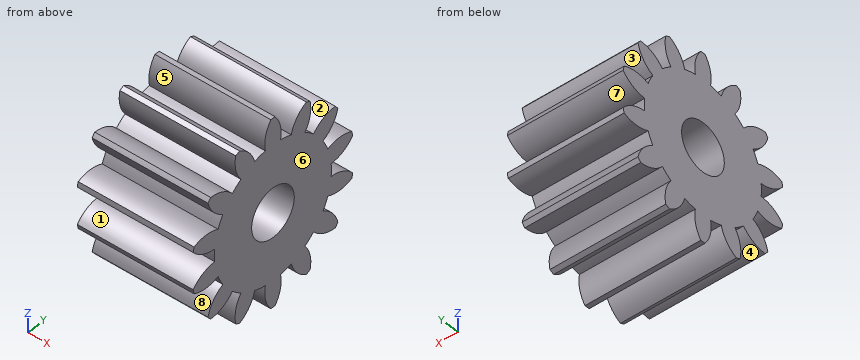
```python
from build123d import *

# Parameters (mm, degrees)
SPUR_START             = 15.199213342
SPUR_GEAR_AM_OUTLINE_R = 2.5
SPUR_GEAR_AM_DEPTH     = 5
SKETCH9_R              = 2.5
SKETCH9_R_2            = 1.05
BOSS_EXTRUDE1_DEPTH    = 5


# Read off the part's stored shape, not the designer's step: spur gear_am
with BuildPart() as part:
    # spur gear_am outline → spur gear_am (new body)
    with BuildSketch(Plane.YZ.offset(SPUR_START)):
        with BuildLine():
            ThreePointArc((2.747947228, -4.643773619), (2.654088149, -4.687486435), (2.561391914, -4.733613923))
            ThreePointArc((2.561391914, -4.733613923), (2.561783739, -5.337982285), (2.816889806, -5.88587111))
            ThreePointArc((2.816889806, -5.88587111), (2.597713415, -6.044378226), (2.394409068, -6.222788256))
            ThreePointArc((2.394409068, -6.222788256), (1.9170234, -5.852161498), (1.327895004, -5.717294884))
            ThreePointArc((1.327895004, -5.717294884), (1.262297175, -5.797402699), (1.198794721, -5.879181519))
            ThreePointArc((1.198794721, -5.879181519), (1.461373347, -6.423528591), (1.928936024, -6.806472991))
            ThreePointArc((1.928936024, -6.806472991), (1.800238579, -7.04438004), (1.694476903, -7.293332374))
            ThreePointArc((1.694476903, -7.293332374), (1.103558354, -7.166539081), (0.514255579, -7.300641692))
            ThreePointArc((0.514255579, -7.300641692), (0.489911456, -7.401278171), (0.468180222, -7.502511024))
            ThreePointArc((0.468180222, -7.502511024), (0.940938733, -7.879022193), (1.528351497, -8.021175333))
            ThreePointArc((1.528351497, -8.021175333), (1.515623105, -8.291361907), (1.528351497, -8.56154848))
            ThreePointArc((1.528351497, -8.56154848), (0.940938733, -8.70370162), (0.468180222, -9.080212789))
            ThreePointArc((0.468180222, -9.080212789), (0.489911456, -9.181445642), (0.514255579, -9.28208212))
            ThreePointArc((0.514255579, -9.28208212), (1.103558354, -9.416184732), (1.694476903, -9.289391439))
            ThreePointArc((1.694476903, -9.289391439), (1.800238579, -9.538343772), (1.928936024, -9.776250821))
            ThreePointArc((1.928936024, -9.776250821), (1.461373347, -10.159195221), (1.198794721, -10.703542294))
            ThreePointArc((1.198794721, -10.703542294), (1.262297175, -10.785321114), (1.327895004, -10.865428928))
            ThreePointArc((1.327895004, -10.865428928), (1.9170234, -10.730562315), (2.394409068, -10.359935556))
            ThreePointArc((2.394409068, -10.359935556), (2.597713414, -10.538345587), (2.816889806, -10.696852703))
            ThreePointArc((2.816889806, -10.696852703), (2.561783739, -11.244741528), (2.561391914, -11.84910989))
            ThreePointArc((2.561391914, -11.84910989), (2.654088149, -11.895237378), (2.747947228, -11.938950194))
            ThreePointArc((2.747947228, -11.938950194), (3.220217142, -11.561826343), (3.489517843, -11.020773293))
            ThreePointArc((3.489517843, -11.020773293), (3.750097941, -11.093304726), (4.016342706, -11.14101763))
            ThreePointArc((4.016342706, -11.14101763), (4.024220134, -11.745334779), (4.286092716, -12.290021864))
            ThreePointArc((4.286092716, -12.290021864), (4.389623105, -12.291361906), (4.493153494, -12.290021864))
            ThreePointArc((4.493153494, -12.290021864), (4.755026076, -11.745334779), (4.762903504, -11.14101763))
            ThreePointArc((4.762903504, -11.14101763), (5.029148269, -11.093304726), (5.289728367, -11.020773293))
            ThreePointArc((5.289728367, -11.020773293), (5.559029068, -11.561826343), (6.031298982, -11.938950194))
            ThreePointArc((6.031298982, -11.938950194), (6.125158061, -11.895237378), (6.217854296, -11.84910989))
            ThreePointArc((6.217854296, -11.84910989), (6.217462471, -11.244741528), (5.962356404, -10.696852703))
            ThreePointArc((5.962356404, -10.696852703), (6.181532796, -10.538345587), (6.384837142, -10.359935556))
            ThreePointArc((6.384837142, -10.359935556), (6.86222281, -10.730562315), (7.451351206, -10.865428928))
            ThreePointArc((7.451351206, -10.865428928), (7.516949035, -10.785321114), (7.580451489, -10.703542294))
            ThreePointArc((7.580451489, -10.703542294), (7.317872863, -10.159195221), (6.850310186, -9.776250821))
            ThreePointArc((6.850310186, -9.776250821), (6.979007631, -9.538343772), (7.084769307, -9.289391439))
            ThreePointArc((7.084769307, -9.289391439), (7.675687856, -9.416184732), (8.26499063, -9.28208212))
            ThreePointArc((8.26499063, -9.28208212), (8.289334754, -9.181445642), (8.311065988, -9.080212789))
            ThreePointArc((8.311065988, -9.080212789), (7.838307477, -8.70370162), (7.250894713, -8.56154848))
            ThreePointArc((7.250894713, -8.56154848), (7.263623105, -8.291361907), (7.250894713, -8.021175333))
            ThreePointArc((7.250894713, -8.021175333), (7.838307477, -7.879022193), (8.311065988, -7.502511024))
            ThreePointArc((8.311065988, -7.502511024), (8.289334754, -7.40127817), (8.26499063, -7.300641692))
            ThreePointArc((8.26499063, -7.300641692), (7.675687856, -7.166539081), (7.084769307, -7.293332374))
            ThreePointArc((7.084769307, -7.293332374), (6.979007631, -7.04438004), (6.850310186, -6.806472991))
            ThreePointArc((6.850310186, -6.806472991), (7.317872863, -6.423528591), (7.580451489, -5.879181519))
            ThreePointArc((7.580451489, -5.879181519), (7.516949035, -5.797402699), (7.451351206, -5.717294884))
            ThreePointArc((7.451351206, -5.717294884), (6.86222281, -5.852161498), (6.384837142, -6.222788256))
            ThreePointArc((6.384837142, -6.222788256), (6.181532795, -6.044378226), (5.962356404, -5.88587111))
            ThreePointArc((5.962356404, -5.88587111), (6.217462471, -5.337982285), (6.217854296, -4.733613923))
            ThreePointArc((6.217854296, -4.733613923), (6.125158061, -4.687486435), (6.031298982, -4.643773619))
            ThreePointArc((6.031298982, -4.643773619), (5.559029068, -5.02089747), (5.289728367, -5.56195052))
            ThreePointArc((5.289728367, -5.56195052), (5.029148269, -5.489419087), (4.762903504, -5.441706183))
            ThreePointArc((4.762903504, -5.441706183), (4.755026076, -4.837389034), (4.493153494, -4.292701948))
            ThreePointArc((4.493153494, -4.292701948), (4.389623105, -4.291361906), (4.286092716, -4.292701948))
            ThreePointArc((4.286092716, -4.292701948), (4.024220134, -4.837389034), (4.016342706, -5.441706183))
            ThreePointArc((4.016342706, -5.441706183), (3.750097941, -5.489419087), (3.489517843, -5.56195052))
            ThreePointArc((3.489517843, -5.56195052), (3.220217142, -5.02089747), (2.747947228, -4.643773619))
        make_face()
        with Locations((4.389623105, -8.291361906)):
            Circle(SPUR_GEAR_AM_OUTLINE_R, mode=Mode.SUBTRACT)
    extrude(amount=SPUR_GEAR_AM_DEPTH)

    # Sketch9 → Boss-Extrude1 (add, through all)
    with BuildSketch(Plane(origin=(20.199213342, 0, 0), x_dir=(0, 0, -1), z_dir=(1, 0, 0))):
        with Locations((8.291361906, 4.389623105)):
            Circle(SKETCH9_R)
        with Locations((8.291361906, 4.389623105)):
            Circle(SKETCH9_R_2, mode=Mode.SUBTRACT)
    extrude(amount=-BOSS_EXTRUDE1_DEPTH)


solid = part.part
```
The model under review builds one solid part; all positions refer to its coordinate system, in mm. Face numbers are marked on the shaded views. A direction names the side the tool comes from. Coordinates: 2 decimals unless noted, no trailing zeros. Write each loop counter-clockwise with the first axis right and the second up, starting at its lowest first coordinate (ties: lowest second). Pieces come first, ordered by that corner, then holes.
1) We need section D-D on z = -6. State the section outline as (x, y) points.
2) Machinability: for the marked faces 4, 5, 6, 7 and 8, which of the approach directions +Z, -Z, +X, -X, +Y, -Y give a long, thin tool a straight path to every point of the face, cutting with its end or side? Answer none if there is none.
3) We need section B-B on z = -7.75. State the section outline as (x, y) points, then the cut area to 3 significant figures.
4) We need section A-A on z = -11.25. State the section outline as (x, y) points, then the cut area to 3 significant figures.
5) The part is to be moulded in two halves that separate along Y. For the marked faces 1, 2 and 3, say which applies: pulls with the +Y half, pulls with the -Y half, needs draft (parallel to the pull), parting line crosses it, or undercut.
6) To check wall thickness, follow probe 1 along Z at (x, y) = (15.7, 7); probe 2 along Y at (x, z) = (17.8, -10.5); probe 3 along Y at (x, z) = (16.45, -11.5). State the ranges of each line that lie inside material, in increasing order.
7) We need section C-C on y = 2.25. State the section outline as (x, z) points.
Answer list:
1. outline: (15.2, 1.23) - (20.2, 1.23) - (20.2, 2.16) - (15.2, 2.16) - close; (15.2, 2.65) - (20.2, 2.65) - (20.2, 6.12) - (15.2, 6.12) - close; (15.2, 6.62) - (20.2, 6.62) - (20.2, 7.55) - (15.2, 7.55) - close
2. face 4: -Z, +X, -X
2. face 5: +X, -X
2. face 6: +Z, -Z, +X, +Y, -Y
2. face 7: +X, -X, +Y
2. face 8: +X, -X, -Y
3. outline: (15.2, 0.73) - (20.2, 0.73) - (20.2, 3.49) - (15.2, 3.49) - close; (15.2, 5.29) - (20.2, 5.29) - (20.2, 8.05) - (15.2, 8.05) - close
3. area: 27.6 mm2
4. outline: (15.2, 2.56) - (20.2, 2.56) - (20.2, 3.41) - (15.2, 3.41) - close; (15.2, 4) - (20.2, 4) - (20.2, 4.78) - (15.2, 4.78) - close; (15.2, 5.37) - (20.2, 5.37) - (20.2, 6.22) - (15.2, 6.22) - close
4. area: 12.4 mm2
5. face 1: pulls with the -Y half
5. face 2: undercut
5. face 3: pulls with the +Y half
6. probe 1: z = -10.79 to -9.86, -9.49 to -7.09, -6.72 to -5.8
6. probe 2: y = 1.26 to 2.26, 2.55 to 6.23, 6.52 to 7.52
6. probe 3: y = 2.53 to 3.27, 3.99 to 4.79, 5.51 to 6.25
7. outline: (15.2, -10.51) - (20.2, -10.51) - (20.2, -6.07) - (15.2, -6.07) - close
